from build123d import *

# Parameters (mm, degrees)
ESQUISSE1_R             = 11.25
BOSS_EXTRU_1_DEPTH      = 13.75
ESQUISSE3_W             = 13.788582234
ESQUISSE3_H             = 13.788582234
ENL_V_MAT_EXTRU_3_DEPTH = 10


with BuildPart() as part:
    # Esquisse1 → Boss.-Extru.1 (new, symmetric)
    with BuildSketch(Plane(origin=(0, 0, 0), x_dir=(1, 0, 0), z_dir=(0, 1, 0))):
        with Locations(Location((0, 0, 0), (0, 0, 270))):
            Circle(ESQUISSE1_R)
    extrude(amount=BOSS_EXTRU_1_DEPTH, both=True)

    # Esquisse3 → Enlèv. mat.-Extru.3 (cut)
    with BuildSketch(Plane(origin=(0, 13.75, 0), x_dir=(1, 0, 0), z_dir=(0, 1, 0))):
        Rectangle(ESQUISSE3_W, ESQUISSE3_H)
    enl_v_mat_extru_3 = extrude(amount=-ENL_V_MAT_EXTRU_3_DEPTH, mode=Mode.SUBTRACT)

    # Symétrie1: Enlèv. mat.-Extru.3 across plane
    add(enl_v_mat_extru_3.mirror(Plane.ZX), mode=Mode.SUBTRACT)


solid = part.part
Part model, mm, in its own coordinate system. A direction names the side the tool comes from. Coordinates: 2 decimals unless noted, no trailing zeros. Loops run counter-clockwise (first coordinate to the right, second up) from the corner with the lowest first, then second, coordinate; pieces in that order, holes last. Notation, with made-up numbers: (74, 51) -> (79, 51) arc R14 ccw to (79, 75) -> close; hole circle Ø10 at (88, 45). An arc over 180 degrees is marked (long way). Use a Markdown table: item, result. Add a question column.
Item 1: Band-saw the part on C-C on y = 10. Write the cut outline in (x, z).
Item 2: Pull direction X, two halves, no side cores. Call faces 1 (the flat face through (6.894, 9, 0)), 2 (the cylindrical face through (-4.31, 0.19, 10.39)), 3 (the flat face through (0.2, 13.75, 7.3)): +X half, -X half, draft (parallel to the pull), parting line (faces both ways), or undercut.
Item 3: Band-saw the part on B-B on z = 0. Write the cut outline in (x, y), plus the area to 3 significant figures.
Item 4: Probe probe 1 along Z at (x, y) = (-1.75, -5.75); probe 2 along Z at (x, y) = (-1, 8.75). List the from-to ranges inside material, lowest first.
Item 5: Flat gauge pins, fed straight in: P1, Ø8, axis at y = 9.5, z = 8.5, coming from the -X side; P2, Ø3, axis at y = -9, z = 2.5, coming from the -X side; P3, Ø5, axis at x = -8.5, y = -4, coming from the +Z side. Where does each tip first touch, or does it go through?
Item 6: Band-saw the part on D-D on y = -0.75. Write the cut outline in (x, z).
Item 7: Which spindle directions (+Z, -Z, +X, -X, +Y, -Y) get a long thin tool onto all of the face, cutting with end or side? Do faces 4 (the flat face through (0, -3.75, 0)), 5 (the flat face through (-6.894, 9, 0)), 6 (the flat face through (0.2, -13.75, 7.3)). Say none if no direction does.
Item 8: Band-saw the part on A-A on x = 0. Write the cut outline in (y, z), plus the area to 3 significant figures.
Geometry says:
| question | item | result |
|---|---|---|
| 1 | outline | circle Ø22.5 at (0, 0); hole (-6.89, -6.89) -> (6.89, -6.89) -> (6.89, 6.89) -> (-6.89, 6.89) -> close |
| 2 | face 1 | undercut |
| 2 | face 2 | parting line |
| 2 | face 3 | draft |
| 3 | outline | (-11.25, -13.75) -> (-6.89, -13.75) -> (-6.89, -3.75) -> (6.89, -3.75) -> (6.89, -13.75) -> (11.25, -13.75) -> (11.25, 13.75) -> (6.89, 13.75) -> (6.89, 3.75) -> (-6.89, 3.75) -> (-6.89, 13.75) -> (-11.25, 13.75) -> close |
| 3 | area | 343 mm² |
| 4 | probe 1 | -11.11 to -6.89, 6.89 to 11.11 |
| 4 | probe 2 | -11.21 to -6.89, 6.89 to 11.21 |
| 5 | P1 | x = -10.31 |
| 5 | P2 | x = -11.21 |
| 5 | P3 | z = 9.52 |
| 6 | outline | circle Ø22.5 at (0, 0) |
| 7 | face 4 | -Y |
| 7 | face 5 | +Y |
| 7 | face 6 | +Z, -Z, +X, -X, -Y |
| 8 | outline | (-13.75, -11.25) -> (13.75, -11.25) -> (13.75, -6.89) -> (3.75, -6.89) -> (3.75, 6.89) -> (13.75, 6.89) -> (13.75, 11.25) -> (-13.75, 11.25) -> (-13.75, 6.89) -> (-3.75, 6.89) -> (-3.75, -6.89) -> (-13.75, -6.89) -> close |
| 8 | area | 343 mm² |
